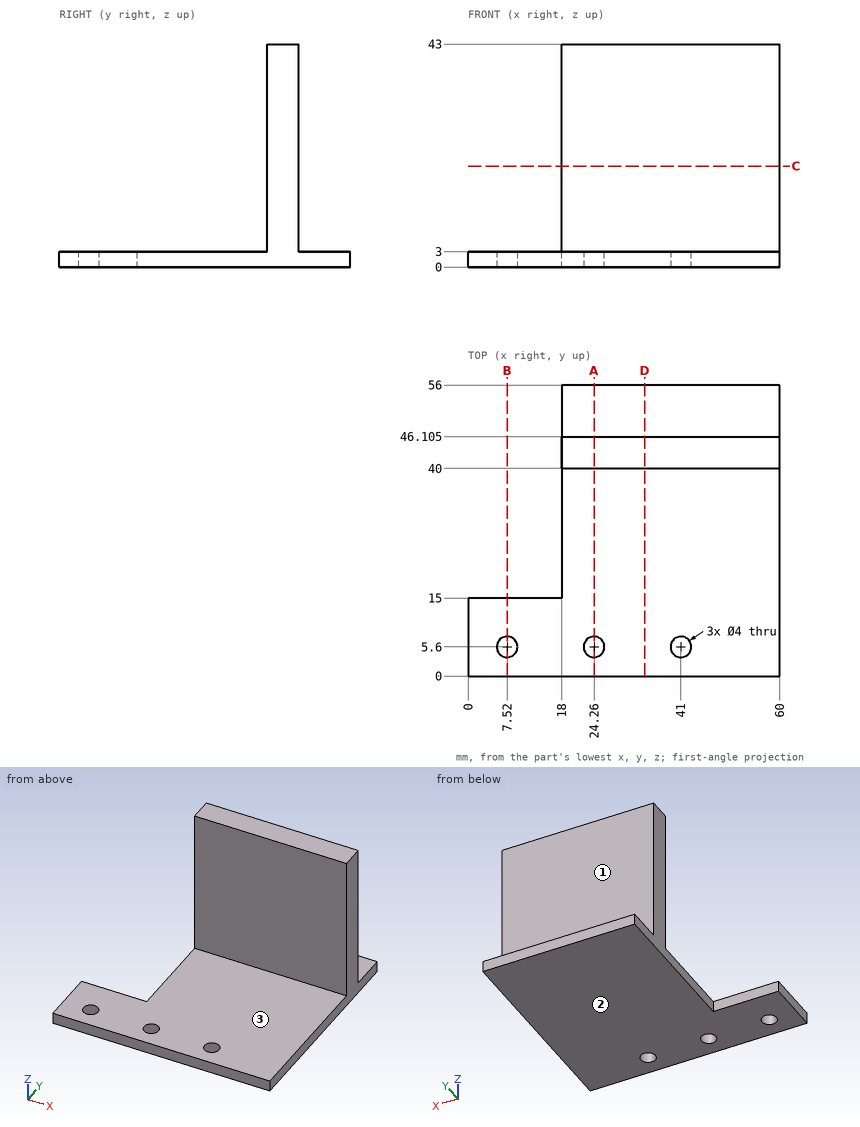
The drawing under review shows one solid part. Ordinate dimensions are in mm from its lowest x, y, z. A direction names the side the tool comes from. Coordinates: 2 decimals unless noted, no trailing zeros. Loops run counter-clockwise (first coordinate to the right, second up) from the corner with the lowest first, then second, coordinate; pieces in that order, holes last.
Item 1: Clearance check with flat-ended pins moving along their axes: pin 1 (12 mm diameter, centred on x = 13, y = 26.5, fed in from +Z); pin 2 (1 mm diameter, centred on x = 34, z = 6, fed in from -Y); pin 3 (2.5 mm diameter, centred on x = 41, y = 5.6, fed in from +Z); pin 4 (0.9 mm diameter, centred on x = 10, z = 2, fed in from +Y). State where each tip first meets the part, or that it passes through.
Completed:
pin 1: stops at z = 3
pin 2: stops at y = 40
pin 3: passes through
pin 4: stops at y = 15
Item 2: Add section A-A (x = 24.26). Write out the cut boundary in (y, z) (1 decimal), and give its area (3 significant figures).
Completed:
outline: (0, 0) - (3.6, 0) - (3.6, 3) - (0, 3) - close; (7.6, 0) - (56, 0) - (56, 3) - (46.1, 3) - (46.1, 43) - (40, 43) - (40, 3) - (7.6, 3) - close
area: 400 mm2
Item 3: Add section B-B (x = 7.52). Write out the cut boundary in (y, z).
Completed:
outline: (0, 0) - (3.6, 0) - (3.6, 3) - (0, 3) - close; (7.6, 0) - (15, 0) - (15, 3) - (7.6, 3) - close
Item 4: For the marked faces 1, 2 and 3, list the 3-axis set-ups (+Z, -Z, +X, -X, +Y, -Y) from which the entire face can be reached by the end or side of a thin tool; tool diameter is ignored.
Completed:
face 1: +Z, +X, -X, +Y
face 2: -Z, +X, -X, +Y, -Y
face 3: +Z, +X, -X, -Y
Item 5: Wall thickness on L1, parallel to X at y = 5, z = 1; L2, parallel to Y at x = 41, z = 1; L3, parallel to Y at x = 50.5, z = 14.5 (1 decimal): over which ranges is each line inside the solid? List them lowest first.
Completed:
L1: x = 0 to 5.61, 9.43 to 22.35, 26.17 to 39.09, 42.91 to 60
L2: y = 0 to 3.6, 7.6 to 56
L3: y = 40 to 46.1
Item 6: Add section D-D (x = 34). Write out the cut boundary in (y, z) (1 decimal).
Completed:
outline: (0, 0) - (56, 0) - (56, 3) - (46.1, 3) - (46.1, 43) - (40, 43) - (40, 3) - (0, 3) - close
Item 7: Add section C-C (z = 19.5). Write out the cut boundary in (x, y) (1 decimal), and give its area (3 significant figures).
Completed:
outline: (18, 40) - (60, 40) - (60, 46.1) - (18, 46.1) - close
area: 256 mm2
